Read the model definition and answer for the solid it produces. Units are mm, in the model's axes. A direction names the side the tool comes from. Give positions to 0.01 mm unless a question says otherwise; leave off trailing zeros. Write each loop counter-clockwise with the first axis right and the second up, starting at its lowest first coordinate (ties: lowest second). Pieces come first, ordered by that corner, then holes. Notation, with made-up numbers: (-31, 64.25) -> (-2, 64.25) arc R20 cw to (-2, 75.25) -> close; hole circle Ø6 at (63.25, 11). An arc over 180 degrees is marked (long way). Answer as CSV lines item,"result". Start each with the question number.
1. A tool of negligible diameter and unlimited length cuts with its end or side. For faces 4 (the flat face through (-21, -2, 5)), 5 (the flat face through (-23, -2, 0)), 6 (the flat face through (-5, -2, -2)), from which of +Z, -Z, +X, -X, +Y, -Y can it reach the whole face along a straight path? Write none if from no direction.
2. The part is cut by section C-C, the plane z = 2.5. Determine the outline of the cut face in (x, y), and give its area (3 significant figures).
3. Given pin 1 (2 mm diameter, centred on x = -14, y = -0.5, fed in from +Z); pin 2 (2.5 mm diameter, centred on x = -17, y = -2, fed in from -Z); pin 3 (1.5 mm diameter, centred on y = -1, z = 15.5, fed in from +X), each flat-ended and moving along its own axis, determine where each tip first touches the part or whether it passes through.
4. The part is cut by section B-B, the plane y = -1.1. Determine the outline of the cut face in (x, z).
5. The part is cut by section D-D, the plane x = -31.5. Determine the outline of the cut face in (y, z).
6. For a pull along X with two mould halves and no side action, classify faces 1 (the flat face through (-5, -2, 7)), 2 (the cylindrical face through (-8.925, -2.465, 6.434)), 3 (the flat face through (0, -2, 2)) as pulls with the +X half, pulls with the -X half, needs draft (parallel to the pull), parting line crosses it, or undercut.
7. Find the intervals of material crossed by line 1 (Z direction, x = -5, y = -3.6); line 2 (Z direction, x = -16, y = -3.95); line 3 (X direction, y = -4.7, z = 5.75), in increasing order.
8. The part is cut by section A-A, the plane x = -5. Determine the outline of the cut face in (y, z).
from build123d import *

# Parameters (mm, degrees)
F0_R        = 1.5
F1_DEPTH    = 5
F2_T1_DEPTH = 20
F2_T3_DEPTH = 19.1421356237


# Not quite as in the source:
# - a fillet or chamfer that OpenCascade refuses, or shapes differently, is made with other operations: its cross-section is extruded or revolved along the edge and cut away or added


with BuildPart() as f1:
    # F0 (on Front) → F1 (new body)
    with BuildSketch(Plane.XZ):
        with BuildLine():
            Line((-38, 0), (-10, 0))
            Line((-10, 0), (-10, -2))
            Line((-10, -2), (0, -2))
            Line((0, -2), (0, 0))
            Line((0, 0), (0, 5))
            Line((0, 5), (0, 7))
            Line((0, 7), (-10, 7))
            Line((-10, 7), (-10, 5))
            Line((-10, 5), (-32.1208064244, 5))
            Line((-32.1208064244, 5), (-36, 27))
            ThreePointArc((-36, 27), (-37, 28), (-38, 27))
            Line((-38, 27), (-38, 0))
        make_face()
        with Locations((-5, 2.5)):
            Circle(F0_R, mode=Mode.SUBTRACT)
    extrude(amount=F1_DEPTH)

    # F2: fillet of radius 3 on 5 edges, made by hand

    # F2_s2 → F2_t1 (cut)
    with BuildSketch(Plane.XZ.offset(-7.5)):
        with BuildLine():
            ThreePointArc((-3, 7), (-0.8786796564, 6.1213203436), (0, 4))
            Line((0, 4), (0, 7))
            Line((0, 7), (-3, 7))
        make_face()
        with BuildLine():
            ThreePointArc((0, 1), (-0.8786796564, -1.1213203436), (-3, -2))
            Line((-3, -2), (0, -2))
            Line((0, -2), (0, 1))
        make_face()
        with BuildLine():
            ThreePointArc((-35, 0), (-37.1213203436, 0.8786796564), (-38, 3))
            Line((-38, 3), (-38, 0))
            Line((-38, 0), (-35, 0))
        make_face()
    extrude(amount=F2_T1_DEPTH, mode=Mode.SUBTRACT)

    # F2_s4 → F2_t3 (cut)
    with BuildSketch(Plane.XZ.offset(-7.0710678119)):
        with BuildLine():
            ThreePointArc((-10, 5), (-8.9036236828, 6.4494897428), (-7.1715728753, 7))
            Line((-7.1715728753, 7), (-10, 7))
            Line((-10, 7), (-10, 5))
        make_face()
        with BuildLine():
            ThreePointArc((-7.1715728753, -2), (-8.9036236828, -1.4494897428), (-10, 0))
            Line((-10, 0), (-10, -2))
            Line((-10, -2), (-7.1715728753, -2))
        make_face()
    extrude(amount=F2_T3_DEPTH, mode=Mode.SUBTRACT)


solid = f1.part
Results found:
1,face 4,"+Z, +Y, -Y"
1,face 5,"-Z, -X, +Y, -Y"
1,face 6,"-Z, +X, -X, +Y, -Y"
2,outline,"(-37.96, -5) -> (-6.5, -5) -> (-6.5, 0) -> (-37.96, 0) -> close; (-3.5, -5) -> (0, -5) -> (0, 0) -> (-3.5, 0) -> close"
2,area,"175 mm²"
3,pin 1,"stops at z = 5"
3,pin 2,"stops at z = 0"
3,pin 3,"stops at x = -33.84"
4,outline,"(-38, 3) arc R3 ccw to (-35, 0) -> (-10, 0) arc R3 ccw to (-7.17, -2) -> (-3, -2) arc R3 ccw to (0, 1) -> (0, 4) arc R3 ccw to (-3, 7) -> (-7.17, 7) arc R3 ccw to (-10, 5) -> (-32.12, 5) -> (-36, 27) arc R1 ccw to (-38, 27) -> close; hole circle Ø3 at (-5, 2.5)"
5,outline,"(-5, 0) -> (0, 0) -> (0, 5) -> (-5, 5) -> close"
6,face 1,"needs draft"
6,face 2,"undercut"
6,face 3,"pulls with the +X half"
7,line 1,"z = -2 to 1, 4 to 7"
7,line 2,"z = 0 to 5"
7,line 3,"x = -38 to -32.25, -9.61 to -0.56"
8,outline,"(-5, -2) -> (0, -2) -> (0, 1) -> (-5, 1) -> close; (-5, 4) -> (0, 4) -> (0, 7) -> (-5, 7) -> close"
